from build123d import *

# Parameters (mm, degrees)
BOSS_EXTRUDE1_DEPTH = 0.508
SKETCH2_R           = 1.55
SKETCH2_R_2         = 4
CUT_EXTRUDE1_DEPTH  = 1.6


with BuildPart() as part:
    # Sketch1 → Boss-Extrude1 (new body)
    with BuildSketch(Plane(origin=(0, 0, 0), x_dir=(1, 0, 0), z_dir=(0, 1, 0))):
        with BuildLine():
            Line((-22.5, 15), (22.5, 15))
            ThreePointArc((22.5, 15), (37.5, 0), (22.5, -15))
            Line((22.5, -15), (-22.5, -15))
            ThreePointArc((-22.5, -15), (-37.5, 0), (-22.5, 15))
        make_face()
    extrude(amount=BOSS_EXTRUDE1_DEPTH)

    # Sketch2 → Cut-Extrude1 (cut)
    with BuildSketch(Plane(origin=(0, 0.508, 0), x_dir=(1, 0, 0), z_dir=(0, 1, 0))):
        with Locations(Location((0, 8.5, 0), (0, 0, 270))):
            Circle(SKETCH2_R)
        with Locations(Location((7.361215932, -4.25, 0), (0, 0, 270))):
            Circle(SKETCH2_R)
        with Locations(Location((-7.361215932, -4.25, 0), (0, 0, 270))):
            Circle(SKETCH2_R)
        with Locations(Location((0, 0, 0), (0, 0, 270))):
            Circle(SKETCH2_R_2)
    extrude(amount=-CUT_EXTRUDE1_DEPTH, mode=Mode.SUBTRACT)


solid = part.part
Source: CAD feature listing. Evaluate the final solid. Frame: model axes, mm. Round coordinates to 2 decimals unless told otherwise and drop trailing zeros. Loops run counter-clockwise (first coordinate to the right, second up) from the corner with the lowest first, then second, coordinate; pieces in that order, holes last. Notation, with made-up numbers: (-11.5, 27.25) - (7.5, 27.25) arc R16 ccw to (7.5, 52.25) - close; hole circle Ø8 at (-22, 54.25). An arc over 180 degrees is marked (long way). Write item = value, one per line. Start each with the question number.
(1) Ray query, line 1 along X through (y, z) = (0.3, 4.25); line 2 along X through (y, z) = (0.3, 0); line 3 along X through (y, z) = (0.35, -7.5). Return the intervals inside material, ascending. Write a range as from..to.
(2) Section query C-C, the plane y = 0.3. Output: boundary loops of the cut face in (x, z), plus the area to 3 significant figures.
(3) Pin query (flat end, axial travel): pin 1 (6.5 mm diameter, centred on x = 0, z = 0, fed in from -Y). Return the tip coordinate at first contact, or that it passes through.
(4) Pull-direction query (Z, two-part tool) for faces 1 (the face through (6.42, 0.26, 3.02)), 2 (the face through (-0.94, 0.26, -9.73)), 3 (the face through (1, 0, 6)), 4 (the face through (37.496, 0.25, -0.33)); classes: +Z half, -Z half, draft (parallel to the pull), parting line (faces both ways), or undercut.
(5) Section query D-D, the plane z = -12. Output: boundary loops of the cut face in (x, y), plus the area to 3 significant figures.
(6) Section query A-A, the plane x = 0. Output: boundary loops of the cut face in (y, z), plus the area to 3 significant figures.
(7) Section query B-B, the plane z = 0. Output: boundary loops of the cut face in (x, y).
Conclusion:
q1.line_1 = -36.89..-8.91, -5.81..5.81, 8.91..36.89
q1.line_2 = -37.5..-4, 4..37.5
q1.line_3 = -35.49..-1.18, 1.18..35.49
q2.outline = (-22.5, -15) - (22.5, -15) arc R15 ccw to (22.5, 15) - (-22.5, 15) arc R15 ccw to start; hole circle Ø3.1 at (-7.36, 4.25); hole circle Ø8 at (0, 0); hole circle Ø3.1 at (0, -8.5); hole circle Ø3.1 at (7.36, 4.25)
q2.area = 1,980 mm2
q3.pin_1 = through
q4.face_1 = undercut
q4.face_2 = undercut
q4.face_3 = draft
q4.face_4 = parting line
q5.outline = (-31.5, 0) - (31.5, 0) - (31.5, 0.51) - (-31.5, 0.51) - close
q5.area = 32.0 mm2
q6.outline = (0, -15) - (0.51, -15) - (0.51, -10.05) - (0, -10.05) - close; (0, -6.95) - (0.51, -6.95) - (0.51, -4) - (0, -4) - close; (0, 4) - (0.51, 4) - (0.51, 15) - (0, 15) - close
q6.area = 9.60 mm2
q7.outline = (-37.5, 0) - (-4, 0) - (-4, 0.51) - (-37.5, 0.51) - close; (4, 0) - (37.5, 0) - (37.5, 0.51) - (4, 0.51) - close
